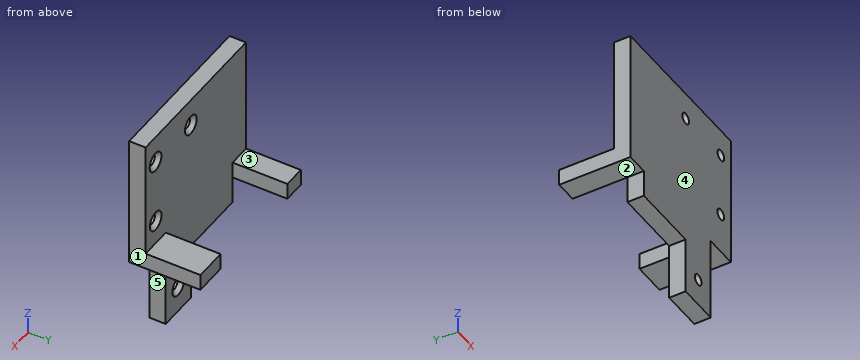
```python
from build123d import *

# Parameters (mm, degrees)
SKETCH1_W           = 60
SKETCH1_H           = 80
BOSS_EXTRUDE1_DEPTH = 6
SKETCH2_R           = 2
CUT_EXTRUDE1_DEPTH  = 51.358713248
SKETCH3_W           = 12
SKETCH3_H           = 6
SKETCH3_W_2         = 8
BOSS_EXTRUDE2_DEPTH = 20
CHAMFER1_SIZE       = 1.5


with BuildPart() as part:
    # Sketch1 → Boss-Extrude1 (new body)
    with BuildSketch(Plane(origin=(0, 0, 0), x_dir=(1, 0, 0), z_dir=(0, 1, 0))):
        Rectangle(SKETCH1_W, SKETCH1_H)
    extrude(amount=BOSS_EXTRUDE1_DEPTH)

    # Sketch2 → Cut-Extrude1 (cut, through all)
    with BuildSketch(Plane(origin=(0, 6, 0), x_dir=(1, 0, 0), z_dir=(0, 1, 0))):
        with Locations(Location((3, -30, 0), (0, 0, 270))):
            Circle(SKETCH2_R)
        with Locations(Location((24.071589502, -30, 0), (0, 0, 270))):
            Circle(SKETCH2_R)
        with Locations(Location((24, -6, 0), (0, 0, 270))):
            Circle(SKETCH2_R)
        with Locations(Location((10.5, 30, 0), (0, 0, 270))):
            Circle(SKETCH2_R)
        Polygon((-40.891606185, 9), (-22, 9), (-22, 19), (3, 19), (3, 40), (18, 40), (18, 9), (35.945141675, 9), (35.945141675, 57.336722716), (-40.891606185, 57.336722716), align=None)
    extrude(amount=-CUT_EXTRUDE1_DEPTH, mode=Mode.SUBTRACT)

    # Sketch3 → Boss-Extrude2 (add)
    with BuildSketch(Plane(origin=(0, 6, 0), x_dir=(1, 0, 0), z_dir=(0, 1, 0))):
        with Locations((24, 6)):
            Rectangle(SKETCH3_W, SKETCH3_H)
        with Locations((-26, 6)):
            Rectangle(SKETCH3_W_2, SKETCH3_H)
    extrude(amount=BOSS_EXTRUDE2_DEPTH)

    # Chamfer1
    chamfer1_edges = [part.edges().sort_by_distance(p)[0] for p in [
        (3, 6, 28),
        (24.071589502, 6, 28),
        (24, 6, 4),
        (10.5, 6, -32),
    ]]
    chamfer(chamfer1_edges, length=CHAMFER1_SIZE)


solid = part.part
```
Work out the finished part from the listing and answer in its coordinate system (mm). Face numbers are marked on the shaded views. A direction names the side the tool comes from. Give positions to 0.01 mm unless a question says otherwise; leave off trailing zeros. Write each loop counter-clockwise with the first axis right and the second up, starting at its lowest first coordinate (ties: lowest second). Pieces come first, ordered by that corner, then holes. Notation, with made-up numbers: (37, 26) - (88, 26) arc R12 ccw to (88, 46) - close; hole circle Ø11 at (-8, -33). An arc over 180 degrees is marked (long way). Use one line per item in the form item = value.
1. Each of these flat-tipped pins is pushed along its axis until it touches: pin 1 Ø3.5 at (x, y) = (21.5, 11) entering from +Z; pin 2 Ø8 at (x, z) = (2.5, -28) entering from +Y; pin 3 Ø6.5 at (x, z) = (24, 6) entering from +Y. Where does it stop, or does it pass through?
Filled in:
pin_1 = -3
pin_2 = 6
pin_3 = 5.75
2. For the marked faces 1, 2, 3, 4 and 5, determine the directions among +Z, -Z, +X, -X, +Y, -Y from which every point of the face is accessible in a straight line to the end or side of a thin tool.
Filled in:
face_1 = +Z, -Z, +X, +Y, -Y
face_2 = -Z, -X, +Y, -Y
face_3 = +Z, +X, -X, +Y
face_4 = +Z, -Z, +X, -X, -Y
face_5 = -Z, +X, +Y, -Y
3. A cutting plane is placed at B-B (y = 8). Write down the section's boundary in (x, z), and give its area (3 significant figures).
Filled in:
outline = (-30, -9) - (-22, -9) - (-22, -3) - (-30, -3) - close; (18, -9) - (30, -9) - (30, -3) - (18, -3) - close
area = 120 mm^2
4. Consider L1, parallel to X at y = 1.3, z = 30; L2, parallel to X at y = 2.05, z = -30; L3, parallel to Z at x = 24, y = 6.5. Determine where each line is inside the solid, lowest interval first.
Filled in:
L1 = -30 to 1, 5 to 22.07, 26.07 to 30
L2 = 3 to 8.5, 12.5 to 18
L3 = -9 to -3
5. A cutting plane is placed at D-D (z = -5.5). Write down the section's boundary in (x, y), and give its area (3 significant figures).
Filled in:
outline = (-30, 0) - (30, 0) - (30, 26) - (18, 26) - (18, 6) - (-22, 6) - (-22, 26) - (-30, 26) - close
area = 760 mm^2
6. A cutting plane is placed at C-C (x = 10.5). Write down the section's boundary in (y, z).
Filled in:
outline = (0, -40) - (6, -40) - (6, -33.5) - (4.5, -32) - (0, -32) - close; (0, -28) - (4.5, -28) - (6, -26.5) - (6, 40) - (0, 40) - close
7. A cutting plane is placed at A-A (z = 6). Write down the section's boundary in (x, y).
Filled in:
outline = (-30, 0) - (22, 0) - (22, 4.5) - (20.5, 6) - (-30, 6) - close; (26, 0) - (30, 0) - (30, 6) - (27.5, 6) - (26, 4.5) - close
